Source: CAD feature listing. Evaluate the final solid. Frame: model axes, mm. A direction names the side the tool comes from. Coordinates: 2 decimals unless noted, no trailing zeros. Write each loop counter-clockwise with the first axis right and the second up, starting at its lowest first coordinate (ties: lowest second). Pieces come first, ordered by that corner, then holes. Notation, with made-up numbers: (-20.75, 11.5) -> (30.25, 11.5) arc R21 cw to (30.25, 41.5) -> close; hole circle Ø2 at (-17, -13). An arc over 180 degrees is marked (long way). One line per item, written item: value. Start each with the question number.
1. First-contact query: P1, Ø1, axis at x = 1.5, y = -1.5, coming from the -Z side; P2, Ø3, axis at y = 2, z = -2, coming from the +X side; P3, Ø2.5, axis at y = 0, z = 0, coming from the -X side; P4, Ø0.5, axis at x = -1, z = 0, coming from the -Y side. Flat tips, straight axial feed; report the tip coordinate or a pass-through.
2. Mould query, pull axis Y, two halves, no side actions, for faces 1 (the conical face through (-1.7, -0.8, 1.5)), 2 (the cylindrical face through (0.54, -3.64, -2.79)), 3 (the flat face through (-0.93, -0.8, 1.37)), 4 (the flat face through (29.312, 0, 0)). Classes: released by +Y, released by -Y, zero draft, split by the parting line, or undercut.
3. Line query: line 1 (X direction, y = -0.5, z = 1.5); line 2 (X direction, y = -2.25, z = 2); line 3 (Z direction, x = 14.5, y = 0.25). Output: solid intervals per line, ascending.
4. Access query for faces 5 (the flat face through (-1.829, 0, 2)), 6 (the flat face through (0, 0, 0)), 7 (the flat face through (0.737, -2, -2)). Directions: +Z, -Z, +X, -X, +Y, -Y. A direction counts if a zero-diameter tool reaches every point of the face in a straight line with its end or side. Return the directions, or none.
5. Section query A-A, the plane x = 3. Output: boundary loops of the cut face in (y, z), and give its area (3 significant figures).
from build123d import *

# Parameters (mm, degrees)
CUT_EXTRUDE1_DEPTH = 1.8288


with BuildPart() as part:
    # Sketch1 → Revolve1 (revolve)
    with BuildSketch(Plane.XY):
        with BuildLine():
            Line((0, 0), (29.3116, 0))
            Line((29.3116, 0), (29.3116, 2.413))
            Line((29.3116, 2.413), (0.7366, 2.413))
            Line((0.7366, 2.413), (0.7366, 4.5847))
            Line((0.7366, 4.5847), (0.3556, 4.5847))
            ThreePointArc((0.3556, 4.5847), (-0.901703741, 3.66491926), (-1.8288, 2.413))
            Line((-1.8288, 2.413), (-1.8288, 1.8288))
            Line((-1.8288, 1.8288), (0, 0))
        make_face()
    revolve(axis=Axis((0, 0, 0), (1, 0, 0)))

    # Sketch2 → Cut-Extrude1 (cut)
    with BuildSketch(Plane.ZY.offset(1.8288)):
        Polygon((1.833087105, 0), (0.916543552, 1.5875), (-0.916543552, 1.5875), (-1.833087105, 0), (-0.916543552, -1.5875), (0.916543552, -1.5875), align=None)
    extrude(amount=-CUT_EXTRUDE1_DEPTH, mode=Mode.SUBTRACT)


solid = part.part
Computed values:
1. P1: stops at z = -2.2
1. P2: stops at x = 29.31
1. P3: stops at x = 0
1. P4: stops at y = -3.81
2. face 1: undercut
2. face 2: split by the parting line
2. face 3: undercut
2. face 4: zero draft
3. line 1: x = 0 to 29.31
3. line 2: x = -1.46 to 0.74
3. line 3: z = -2.4 to 2.4
4. face 5: +Z, -Z, -X, +Y, -Y
4. face 6: -X
4. face 7: +X
5. outline: circle Ø4.83 at (0, 0)
5. area: 18.3 mm²
